```python
from build123d import *

# Parameters (mm, degrees)
SKETCH_W        = 60
SKETCH_H        = 60
PAD_DEPTH       = 11.15
SKETCH001_R     = 2.1
SKETCH001_R_2   = 3.2
POCKET_DEPTH    = 12
SKETCH002_R     = 4.2
POCKET001_DEPTH = 3.6
FILLET_R        = 4
CHAMFER_SIZE    = 0.4
CHAMFER001_SIZE = 0.6


with BuildPart() as part:
    # Sketch → Pad (new body)
    with BuildSketch(Plane.XY):
        with Locations((30, 30)):
            Rectangle(SKETCH_W, SKETCH_H)
    extrude(amount=PAD_DEPTH)

    # Sketch001 (on Face6 of Pad) → Pocket (cut)
    with BuildSketch(Plane.XY.offset(11.15)):
        with Locations((15, 35)):
            Circle(SKETCH001_R)
        with Locations((45, 35)):
            Circle(SKETCH001_R)
        with Locations((15, 25)):
            Circle(SKETCH001_R)
        with Locations((45, 25)):
            Circle(SKETCH001_R)
        with Locations((10, 50)):
            Circle(SKETCH001_R_2)
        with Locations((50, 50)):
            Circle(SKETCH001_R_2)
        with Locations((10, 10)):
            Circle(SKETCH001_R_2)
        with Locations((50, 10)):
            Circle(SKETCH001_R_2)
    extrude(amount=-POCKET_DEPTH, mode=Mode.SUBTRACT)

    # Sketch002 (on Face5 of Pocket) → Pocket001 (cut)
    with BuildSketch(Plane.XY.offset(11.15)):
        with Locations((15, 35)):
            Circle(SKETCH002_R)
        with Locations((45, 35)):
            Circle(SKETCH002_R)
        with Locations((45, 25)):
            Circle(SKETCH002_R)
        with Locations((15, 25)):
            Circle(SKETCH002_R)
    extrude(amount=-POCKET001_DEPTH, mode=Mode.SUBTRACT)

    # Fillet
    fillet_edges = [part.edges().sort_by_distance(p)[0] for p in [
        (0, 0, 5.575),
        (0, 60, 5.575),
        (60, 60, 5.575),
        (60, 0, 5.575),
    ]]
    fillet(fillet_edges, radius=FILLET_R)

    # Chamfer
    chamfer_edges = [part.edges().sort_by_distance(p)[0] for p in [
        (30, 60, 11.15),
        (1.171573, 58.828427, 11.15),
        (58.828427, 58.828427, 11.15),
        (0, 30, 11.15),
        (60, 30, 11.15),
        (1.171573, 1.171573, 11.15),
        (58.828427, 1.171573, 11.15),
        (30, 0, 11.15),
        (40.8, 35, 11.15),
        (46.8, 50, 11.15),
        (6.8, 50, 11.15),
        (10.8, 35, 11.15),
        (10.8, 25, 11.15),
        (40.8, 25, 11.15),
        (46.8, 10, 11.15),
        (6.8, 10, 11.15),
    ]]
    chamfer(chamfer_edges, length=CHAMFER_SIZE)

    # Chamfer001
    chamfer001_edges = [part.edges().sort_by_distance(p)[0] for p in [
        (30, 60, 0),
        (1.171573, 58.828427, 0),
        (58.828427, 58.828427, 0),
        (0, 30, 0),
        (60, 30, 0),
        (1.171573, 1.171573, 0),
        (58.828427, 1.171573, 0),
        (30, 0, 0),
        (42.9, 25, 0),
        (42.9, 35, 0),
        (46.8, 50, 0),
        (6.8, 50, 0),
        (12.9, 25, 0),
        (12.9, 35, 0),
        (46.8, 10, 0),
        (6.8, 10, 0),
    ]]
    chamfer(chamfer001_edges, length=CHAMFER001_SIZE)


solid = part.part
```
Model file for the job. Use its own axes, mm. A direction names the side the tool comes from. Coordinates: 2 decimals unless noted, no trailing zeros. Loops run counter-clockwise (first coordinate to the right, second up) from the corner with the lowest first, then second, coordinate; pieces in that order, holes last. Notation, with made-up numbers: (7, 43.5) -> (23, 43.5) arc R24 cw to (23, 82.5) -> close; hole circle Ø5 at (62.25, 54.25). An arc over 180 degrees is marked (long way). Answer as a JSON object with one key per item and string values.
Q1. Pull direction X, two halves, no side cores. Call faces 3 (the conical face through (1.3, 58.6, 11)), 4 (the flat face through (30, 0, 6)), 5 (the flat face through (17, 23, 7.55)): released by +X, released by -X, zero draft, split by the parting line, or undercut.
Report:
{"face 3": "released by -X", "face 4": "zero draft", "face 5": "undercut"}
Q2. Probe probe 1 along Y at (x, z) = (15, 5.75); probe 2 along Y at (x, z) = (49, 3.25); probe 3 along X at (y, z) = (36.5, 9.75). List the from-to ranges inside material, lowest first.
Report:
{"probe 1": "y = 0 to 22.9, 27.1 to 32.9, 37.1 to 60", "probe 2": "y = 0 to 6.96, 13.04 to 46.96, 53.04 to 60", "probe 3": "x = 0 to 11.08, 18.92 to 41.08, 48.92 to 60"}
Q3. Flat gauge pins, fed straight in: P1, Ø4, axis at x = 17, y = 34, coming from the +Z side; P2, Ø2.5, axis at x = 45.5, y = 24, coming from the +Z side; P3, Ø8, axis at x = 45.5, y = 25, coming from the +Z side. Where does each tip first touch, or does it go through?
Report:
{"P1": "stops at z = 10.79", "P2": "stops at z = 7.55", "P3": "stops at z = 11.05"}
Q4. Cut at D-D (y = 10). List the corners of the cut face in (x, z).
Report:
{"outline": "(0, 0.6) -> (0.6, 0) -> (6.2, 0) -> (6.8, 0.6) -> (6.8, 10.75) -> (6.4, 11.15) -> (0.4, 11.15) -> (0, 10.75) -> close; (13.2, 0.6) -> (13.8, 0) -> (46.2, 0) -> (46.8, 0.6) -> (46.8, 10.75) -> (46.4, 11.15) -> (13.6, 11.15) -> (13.2, 10.75) -> close; (53.2, 0.6) -> (53.8, 0) -> (59.4, 0) -> (60, 0.6) -> (60, 10.75) -> (59.6, 11.15) -> (53.6, 11.15) -> (53.2, 10.75) -> close"}
Q5. Cut at A-A (y = 25). State how many separate pieces and enclosed holes the cut face has, and give its area (3 significant figures).
Report:
{"separate pieces": "3", "enclosed holes": "0", "area": "544 mm2"}
Q6. 3-axis set-ups, long thin cutter, end or side, ignore diameter. For faces 1 (the cylindrical face through (10.804, 25.185, 9.172)), 2 (the flat face through (30, 30, 0)): which of +Z, -Z, +X, -X, +Y, -Y reach the whole face in a straight line?
Report:
{"face 1": "+Z", "face 2": "-Z, +X, -X, +Y, -Y"}
